Verification items for the finished model (mm, model axes). A direction names the side the tool comes from. Give positions to 0.01 mm unless a question says otherwise; leave off trailing zeros. Order: outer loops, then holes, each group sorted by start corner. A loop starts at its lowest first (then second) coordinate and runs counter-clockwise, first axis right, second up.
(1) Sectioned sample at A-A on x = -297.5. Record the cut outline in (y, z), plus the area to 3 significant figures.
(2) Mould release check, pull along Y, two halves, no side actions. Record for faces 1 (the face through (0, -54, -15)), 2 (the face through (6.261, -428.931, -145.264)), 3 (the face through (5.87, 602.96, 71.61)): pulls with the +Y half, pulls with the -Y half, needs draft (parallel to the pull), parting line crosses it, or undercut.
(3) Scan lines: L1, parallel to Z at x = 5, y = 0; L2, parallel to X at y = 293.5, z = -1; L3, parallel to Y at x = -358, z = 24.5. Record each from-to range of solid material in increasing order.
(4) Sectioned sample at B-B on y = 190.5. Record the cut outline in (x, z), plus the area to 3 significant figures.
(5) Gauge pin test, flat ends, axial feed: pin 1 (4 mm diameter, centred on x = 9.5, y = 46.5, fed in from +Z); pin 2 (2 mm diameter, centred on y = -32.5, z = -28, fed in from -X); pin 3 (8 mm diameter, centred on y = 337, z = -37.5, fed in from -X); pin 4 (6 mm diameter, centred on x = -180, z = 26, fed in from -Y). Record the tip position at first contact, or that the pin passes through.
(6) Access from +Z, -Z, +X, -X, +Y, -Y to the whole of each face (thin tool, end or side, straight path). Record for faces 4 (the face through (5.82, 282.06, -57.46)), 5 (the face through (6.4, 310.9, -62.2)).
```python
from build123d import *

# Parameters (mm, degrees)
F0_W          = 533.4
F0_H          = 76.2
F0_R          = 6.35
F0_W_2        = 76.2
F0_H_2        = 50.8
F1_DEPTH      = 12.7
F3_DEPTH      = 406.4
F3_DEPTH_BACK = 431.8
F5_DEPTH      = 25.4


with BuildPart() as f1:
    # F0 (on Right) → F1 (new body)
    with BuildSketch(Plane.YZ):
        Rectangle(F0_W, F0_H)
        Circle(F0_R, mode=Mode.SUBTRACT)
        with BuildLine():
            Line((-266.7, -38.1), (-266.7, 38.1))
            ThreePointArc((-266.7, 38.1), (-295.8604775462, 32.2996203774), (-320.5815367264, 15.7815367264))
            Line((-320.5815367264, 15.7815367264), (-266.7, -38.1))
        make_face()
        with BuildLine():
            ThreePointArc((342.9, -38.1), (320.5815367264, 15.7815367264), (266.7, 38.1))
            Line((266.7, 38.1), (266.7, -38.1))
            Line((266.7, -38.1), (342.9, -38.1))
        make_face()
        with BuildLine():
            Line((-374.4630734528, -145.8630734528), (-266.7, -38.1))
            Line((-266.7, -38.1), (-320.5815367264, 15.7815367264))
            Line((-320.5815367264, 15.7815367264), (-428.3446101792, -91.9815367264))
            Line((-428.3446101792, -91.9815367264), (-405.8939698766, -114.4321770291))
            ThreePointArc((-405.8939698766, -114.4321770291), (-398.9738020205, -113.0556700582), (-395.053841816, -118.9223050896))
            ThreePointArc((-395.053841816, -118.9223050896), (-395.5372067846, -121.3523448851), (-396.9137137555, -123.4124331502))
            Line((-396.9137137555, -123.4124331502), (-374.4630734528, -145.8630734528))
        make_face()
        with Locations((304.8, -63.5)):
            Rectangle(F0_W_2, F0_H_2)
        with BuildLine():
            ThreePointArc((-428.3446101792, -91.9815367264), (-428.3446101792, -145.8630734528), (-374.4630734528, -145.8630734528))
            Line((-374.4630734528, -145.8630734528), (-396.9137137555, -123.4124331502))
            ThreePointArc((-396.9137137555, -123.4124331502), (-405.8939698766, -123.4124331502), (-405.8939698766, -114.4321770291))
            Line((-405.8939698766, -114.4321770291), (-428.3446101792, -91.9815367264))
        make_face()
    extrude(amount=F1_DEPTH)

    # F2 (on face) → F3 (join, two sides)
    with BuildSketch(Plane.YZ.offset(12.7)) as f3_sk:
        with BuildLine():
            Line((932.9831600189, -41.8606996536), (936.4036917686, -38.1))
            ThreePointArc((936.4036917686, -38.1), (607.84366322, 77.5570236238), (293.0137515068, -71.4744031429))
            Line((293.0137515068, -71.4744031429), (297.0012426376, -76.2937888503))
            ThreePointArc((297.0012426376, -76.2937888503), (607.900564523, 71.9058559585), (932.9831600189, -41.8606996536))
        make_face()
    extrude(amount=F3_DEPTH)
    extrude(f3_sk.sketch, amount=-F3_DEPTH_BACK)

    # F4 (on face) → F5 (cut)
    with BuildSketch(Plane.YZ.offset(12.7)):
        Polygon((266.7, -88.9), (342.9, -88.9), (347.1251726151, -88.7651666999), (347.1251726151, -30.6838881224), (342.6863394703, -32.397700998), (324.4524045918, -48.4607793352), (297.0012426376, -76.2937888503), (266.7, -38.1), align=None)
    extrude(amount=-F5_DEPTH, mode=Mode.SUBTRACT)


solid = f1.part
```
Ans:
1. outline: (293.01, -71.47) - (297, -76.29) arc R452.15 cw to (932.98, -41.86) - (936.4, -38.1) arc R457.77 ccw to start
1. area: 4,010 mm2
2. face 1: needs draft
2. face 2: parting line crosses it
2. face 3: undercut
3. L1: z = -38.1 to -6.35, 6.35 to 38.1
3. L2: x = 0 to 12.7
3. L3: y = 416.48 to 429.47, 835.22 to 846.63
4. outline: (0, -38.1) - (12.7, -38.1) - (12.7, 38.1) - (0, 38.1) - close
4. area: 968 mm2
5. pin 1: stops at z = 38.1
5. pin 2: stops at x = 0
5. pin 3: stops at x = -419.1
5. pin 4: stops at y = 413.69
6. face 4: -Z, +X, -X
6. face 5: -Z, +X, -X, +Y
